CAD build for the part. Positions are in the model's coordinates, mm. Coordinates: 2 decimals unless noted, no trailing zeros. Loops run counter-clockwise (first coordinate to the right, second up) from the corner with the lowest first, then second, coordinate; pieces in that order, holes last.
1) Saw through at B-B, the plane x = 3.25. Write the cut outline in (y, z).
2) Two-plate mould, pull along Z, no slides. Class faces 1 (the cylindrical face through (3.131, 14.074, 9.871)), 2 (the flat face through (3, 20, -3.235)), 3 (the flat face through (6.35, 20, 29)), 4 (the cylindrical face through (3.131, 14.442, 47.708)): +Z half, -Z half, draft (parallel to the pull), parting line (faces both ways), or undercut.
3) Wall check: line 1 along Z through (x, y) = (0.5, 31.5); line 2 along Z through (x, y) = (4.75, 12); line 3 along Y through (x, z) = (4.5, 47). Give the ranges that are in metal, low to high.
4) Pin check, flat tip, straight feed: pin 1 Ø10 at (y, z) = (12.5, 25) entering from -X. Stop position of the tip, or through.
5) Saw through at C-C, the plane y = 33. Give the number of separate pieces and of enclosed holes in the cut face, and give its area (3 significant figures).
6) Saw through at A-A, the plane y = 23. Write the cut outline in (x, z).
```python
from build123d import *

# Parameters (mm, degrees)
SKETCH1_W                           = 63.5
SKETCH1_H                           = 30.48
BOSS_EXTRUDE1_DEPTH                 = 6.35
TAP_DRILL_FOR_6_32_TAP1_D           = 2.7051
TAP_DRILL_FOR_6_32_TAP1_DEPTH       = 6.35
TAP_DRILL_FOR_6_32_TAP1_CSINK_D     = 3.9751
TAP_DRILL_FOR_6_32_TAP1_CSINK_ANGLE = 90
LPATTERN1_COUNT                     = 2
LPATTERN1_PITCH                     = 40.64
LPATTERN1_COUNT_DIR2                = 2
LPATTERN1_PITCH_DIR2                = 10.16


with BuildPart() as part:
    # Sketch1 → Boss-Extrude1 (new body)
    with BuildSketch(Plane(origin=(0, 0, 0), x_dir=(0, 0, -1), z_dir=(1, 0, 0))):
        with Locations((-28.514872299, 20.201128374)):
            Rectangle(SKETCH1_W, SKETCH1_H)
    extrude(amount=BOSS_EXTRUDE1_DEPTH)

    # Tap Drill for #6-32 Tap1
    with Locations(Plane.ZY):
        with Locations((9.464872299, 32.266128374), (47.564872299, 32.266128374)):
            CounterSinkHole(TAP_DRILL_FOR_6_32_TAP1_D / 2, TAP_DRILL_FOR_6_32_TAP1_CSINK_D / 2, depth=TAP_DRILL_FOR_6_32_TAP1_DEPTH, counter_sink_angle=TAP_DRILL_FOR_6_32_TAP1_CSINK_ANGLE)

    # Sketch8 → #5 Clearance Hole1 (revolve, cut)
    with BuildSketch(Plane(origin=(0, 23.60868099, 8.363470458), x_dir=(0, 0, 1), z_dir=(0, 1, 0))):
        Polygon((0, 0), (0, 13.680574487), (1.63195, 12.7), (1.63195, 0), align=None)
    f_5_clearance_hole1 = revolve(axis=Axis((-6.35, 23.60868099, 8.363470458), (1, 0, 0)), mode=Mode.SUBTRACT)

    # LPattern1: 5 Clearance Hole1 2 × 2
    with Locations(*[(0, -j * LPATTERN1_PITCH_DIR2, i * LPATTERN1_PITCH) for i in range(LPATTERN1_COUNT) for j in range(LPATTERN1_COUNT_DIR2) if (i, j) != (0, 0)]):
        add(f_5_clearance_hole1, mode=Mode.SUBTRACT)


solid = part.part
```
Data:
1. outline: (4.96, -3.24) - (35.44, -3.24) - (35.44, 60.26) - (4.96, 60.26) - close; hole circle Ø3.26 at (13.45, 8.36); hole circle Ø3.26 at (13.45, 49); hole circle Ø3.26 at (23.61, 8.36); hole circle Ø3.26 at (23.61, 49); hole circle Ø2.71 at (32.27, 9.46); hole circle Ø2.71 at (32.27, 47.56)
2. face 1: undercut
2. face 2: -Z half
2. face 3: draft
2. face 4: undercut
3. line 1: z = -3.24 to 8.19, 10.74 to 46.29, 48.84 to 60.26
3. line 2: z = -3.24 to 7.61, 9.11 to 48.25, 49.75 to 60.26
3. line 3: y = 4.96 to 31.04, 33.5 to 35.44
4. pin 1: stops at x = 0
5. separate pieces: 3
5. enclosed holes: 0
5. area: 373 mm2
6. outline: (0, -3.24) - (6.35, -3.24) - (6.35, 6.85) - (0, 6.85) - close; (0, 9.88) - (6.35, 9.88) - (6.35, 47.49) - (0, 47.49) - close; (0, 50.52) - (6.35, 50.52) - (6.35, 60.26) - (0, 60.26) - close
